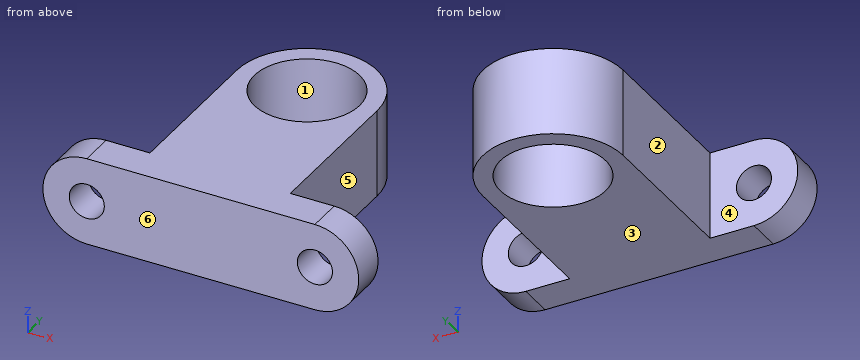
```python
from build123d import *

# Parameters (mm, degrees)
SKETCH1_R           = 152.4
BOSS_EXTRUDE1_DEPTH = 127
SKETCH2_R           = 50.8
BOSS_EXTRUDE2_DEPTH = 101.6


with BuildPart() as part:
    # Sketch1 → Boss-Extrude1 (new, symmetric)
    with BuildSketch(Plane.XY):
        with BuildLine():
            Line((-203.2, -457.2), (203.2, -457.2))
            Line((203.2, -457.2), (203.2, 0))
            ThreePointArc((203.2, 0), (0, 203.2), (-203.2, 0))
            Line((-203.2, 0), (-203.2, -457.2))
        make_face()
        Circle(SKETCH1_R, mode=Mode.SUBTRACT)
    extrude(amount=BOSS_EXTRUDE1_DEPTH, both=True)

    # Sketch2 → Boss-Extrude2 (add)
    with BuildSketch(Plane.XZ.offset(457.2)):
        with BuildLine():
            Line((-203.2, -127), (203.2, -127))
            Line((203.2, -127), (330.2, -127))
            ThreePointArc((330.2, -127), (457.2, 0), (330.2, 127))
            Line((330.2, 127), (203.2, 127))
            Line((203.2, 127), (-203.2, 127))
            Line((-203.2, 127), (-330.2, 127))
            ThreePointArc((-330.2, 127), (-457.2, 0), (-330.2, -127))
            Line((-330.2, -127), (-203.2, -127))
        make_face()
        with Locations((-330.2, 0)):
            Circle(SKETCH2_R, mode=Mode.SUBTRACT)
        with Locations((330.2, 0)):
            Circle(SKETCH2_R, mode=Mode.SUBTRACT)
    extrude(amount=BOSS_EXTRUDE2_DEPTH)


solid = part.part
```
Work out the finished part from the listing and answer in its coordinate system (mm). Face numbers are marked on the shaded views. A direction names the side the tool comes from. Round coordinates to 2 decimals unless told otherwise and drop trailing zeros. Write each loop counter-clockwise with the first axis right and the second up, starting at its lowest first coordinate (ties: lowest second). Pieces come first, ordered by that corner, then holes. Notation, with made-up numbers: (27, 16) - (70, 16) arc R31 cw to (70, 55) - close; hole circle Ø4 at (77, 86.5). An arc over 180 degrees is marked (long way). Return JSON: item names as keys, results as strings. Group by question number.
Q1. The part is cut by section C-C on y = -496.5. Write down the section's boundary in (x, z).
Q2. The mould has two halves that part along X. Classify the marked faces 1, 2 and 3: released by +X, released by -X, zero draft, split by the parting line, or undercut.
Q3. The part is cut by section A-A on x = 0. Write down the section's boundary in (y, z), then the cut area to 3 significant figures.
Q4. For the marked faces 4, 5 and 6, determine the directions among +Z, -Z, +X, -X, +Y, -Y from which every point of the face is accessible in a straight line to the end or side of a thin tool.
Q5. The part is cut by section B-B on z = 18. Write down the section's boundary in (x, y).
Q6. The part is cut by section D-D on y = -25. Write down the section's boundary in (x, z), then the cut area to 3 significant figures.
Q7. Each of these flat-tipped pins is pushed along its axis until it touches: pin 1 Ø1 at (y, z) = (26.5, 31.5) entering from +X; pin 2 Ø4 at (x, z) = (184, -2.5) entering from +Y; pin 3 Ø12 at (y, z) = (-282.5, 29) entering from -X. Where does it stop, or does it pass through?
Q8. Find the intervals of material crossed by L1, parallel to Y at x = 0, z = -15.5; L2, parallel to Z at x = 330, y = -477; L3, parallel to X at y = -318.5, z = -69.5, in increasing order.
Solved:
{
 "1": {"outline": "(-330.2, -127) - (330.2, -127) arc R127 ccw to (330.2, 127) - (-330.2, 127) arc R127 ccw to start; hole circle Ø101.6 at (-330.2, 0); hole circle Ø101.6 at (330.2, 0)"},
 "2": {"face 1": "undercut", "face 2": "released by -X", "face 3": "zero draft"},
 "3": {"outline": "(-558.8, -127) - (-152.4, -127) - (-152.4, 127) - (-558.8, 127) - close; (152.4, -127) - (203.2, -127) - (203.2, 127) - (152.4, 127) - close", "area": "116,000 mm²"},
 "4": {"face 4": "+Z, -Z, -X, +Y", "face 5": "+Z, -Z, +X, +Y", "face 6": "+Z, -Z, +X, -X, -Y"},
 "5": {"outline": "(-455.92, -558.8) - (-377.7, -558.8) - (-377.7, -457.2) - (-455.92, -457.2) - close; (-282.7, -558.8) - (282.7, -558.8) - (282.7, -457.2) - (203.2, -457.2) - (203.2, 0) arc R203.2 ccw to (-203.2, 0) - (-203.2, -457.2) - (-282.7, -457.2) - close; (377.7, -558.8) - (455.92, -558.8) - (455.92, -457.2) - (377.7, -457.2) - close; hole circle Ø304.8 at (0, 0)"},
 "6": {"outline": "(-203.2, -127) - (-150.34, -127) - (-150.34, 127) - (-203.2, 127) - close; (150.34, -127) - (203.2, -127) - (203.2, 127) - (150.34, 127) - close", "area": "26,900 mm²"},
 "7": {"pin 1": "x = 201.53", "pin 2": "y = 90.37", "pin 3": "x = -203.2"},
 "8": {"L1": "-558.8 to -152.4, 152.4 to 203.2", "L2": "-127 to -50.8, 50.8 to 127", "L3": "-203.2 to 203.2"}
}
